Build history of the part. All positions in model axes, mm. Round coordinates to 2 decimals unless told otherwise and drop trailing zeros. Order: outer loops, then holes, each group sorted by start corner. A loop starts at its lowest first (then second) coordinate and runs counter-clockwise, first axis right, second up. Notation, with made-up numbers: M 57.5,30.25 L 93.5,30.25 A20 cw 93.5,36.25 Z; hole C 51,1 d6. An arc over 180 degrees is marked long. One line per item, written item: value. Start each with the question number.
Item 1: Probe L1, parallel to Z at x = 0, y = 1.7; L2, parallel to X at y = 0.65, z = -253; L3, parallel to X at y = 1.55, z = -400. List the from-to ranges inside material, lowest first.
Item 2: Band-saw the part on C-C, the plane z = -122. Write the cut outline in (x, y) (3 decimals).
Item 3: Band-saw the part on B-B, the plane x = 272.5. Write the cut outline in (y, z) (3 decimals), then the cut area to 3 significant figures.
Item 4: Band-saw the part on A-A, the plane y = 0.5. Give the number of separate pieces and of enclosed holes in the cut face, then the cut area to 3 significant figures.
```python
from build123d import *

# Parameters (mm, degrees)
BOSS_EXTRUDE1_DEPTH         = 3.175
F_1_4_0_25_DIAMETER_HOLE1_D = 6.35
F_1_4_CLEARANCE_HOLE1_D     = 6.7564
F_7_0_201_DIAMETER_HOLE1_D  = 5.1054


with BuildPart() as part:
    # Sketch1 → Boss-Extrude1 (new body)
    with BuildSketch(Plane(origin=(0, 0, 0), x_dir=(1, 0, 0), z_dir=(0, 1, 0))):
        Polygon((-462.534, 0), (-215.773, 449.26502653), (215.773, 449.26502653), (462.534, 0), align=None)
    extrude(amount=BOSS_EXTRUDE1_DEPTH)

    # 1/4 (0.25) Diameter Hole1 (through all)
    with Locations(Plane(origin=(0, 3.175, 0), x_dir=(1, 0, 0), z_dir=(0, 1, 0))):
        with Locations((-402.368285269, 83.160171278), (-255.632309055, 350.314795577), (-126.873, 436.56502653), (402.368285269, 83.160171278), (255.632309055, 350.314795577), (126.873, 436.56502653)):
            Hole(F_1_4_0_25_DIAMETER_HOLE1_D / 2)

    # 1/4 Clearance Hole1 (through all)
    with Locations(Plane(origin=(0, 3.175, 0), x_dir=(1, 0, 0), z_dir=(0, 1, 0))):
        with Locations((-376.682, 50.8), (-244.348, 50.8), (-123.952, 250.19), (-185.674, 398.526), (0, 224.79), (376.682, 50.8), (244.348, 50.8), (185.674, 398.526), (123.952, 250.19)):
            Hole(F_1_4_CLEARANCE_HOLE1_D / 2)

    # #7 (0.201) Diameter Hole1 (through all)
    with Locations(Plane(origin=(0, 3.175, 0), x_dir=(1, 0, 0), z_dir=(0, 1, 0))):
        with Locations((34.925, 334.96502653), (-34.925, 334.96502653), (-34.925, 284.16502653), (34.925, 284.16502653)):
            Hole(F_7_0_201_DIAMETER_HOLE1_D / 2)


solid = part.part
```
Output:
1. L1: z = -449.27 to -228.17, -221.41 to 0
1. L2: x = -323.57 to -125.83, -122.08 to 122.08, 125.83 to 323.57
1. L3: x = -242.83 to -188.71, -182.63 to 182.63, 188.71 to 242.83
2. outline: M -395.525,0 L 395.525,0 L 395.525,3.175 L -395.525,3.175 Z
3. outline: M 0,-345.985 L 3.175,-345.985 L 3.175,0 L 0,0 Z
3. area: 1,100 mm²
4. separate pieces: 1
4. enclosed holes: 19
4. area: 304,000 mm²
